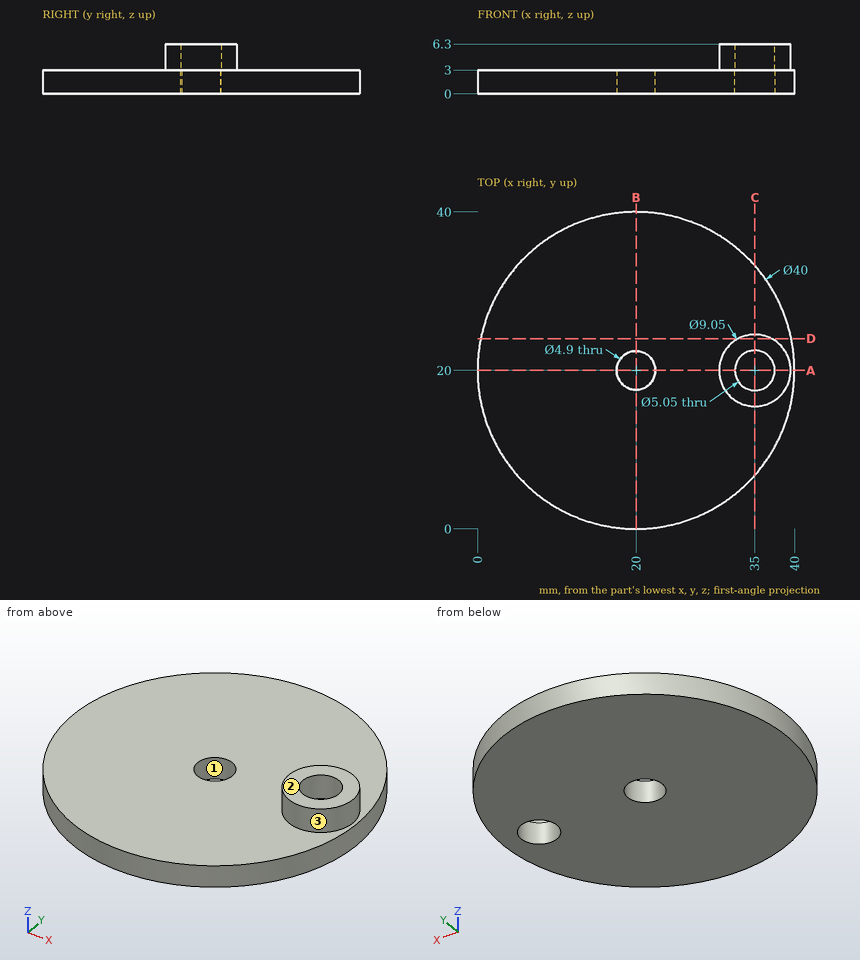
Source: three-view drawing plus pictorial views. Frame: mm from the lowest corner of the part. Give positions to 0.01 mm unless a question says otherwise; leave off trailing zeros. Write each loop counter-clockwise with the first axis right and the second up, starting at its lowest first coordinate (ties: lowest second). Pieces come first, ordered by that corner, then holes.
(1) First-contact query: P1, Ø2, axis at x = 9.5, z = 3, coming from the +Y side; P2, Ø2, axis at x = 6.5, z = 1, coming from the +Y side; P3, Ø2, axis at y = 20.5, z = 4.5, coming from the +X side (3 decimals). Flat tips, straight axial feed; report the tip coordinate or a pass-through.
(2) Cut plane B-B, the plane x = 20. Return loops of the section in (y, z).
(3) Cut plane A-A, the plane y = 20. Return loops of the section in (x, z) (3 decimals).
(4) Mould query, pull axis X, two halves, no side actions, for the marked faces 1, 2 and 3. Classes: released by +X, released by -X, zero draft, split by the parting line, or undercut.
(5) Ray query, line 1 (Y direction, x = 20, z = 1.6); line 2 (X direction, y = 18.5, z = 0.75); line 3 (Z direction, x = 33.5, y = 12.5). Return the intervals inside material, ascending.
(6) Cut plane C-C, the plane x = 35. Return loops of the section in (y, z) (3 decimals), then the cut area to 3 significant figures.
(7) Cut plane D-D, the plane y = 24. Return loops of the section in (x, z), then the cut area to 3 significant figures.
Values follow:
1. P1: stops at y = 37.6
1. P2: stops at y = 35.61
1. P3: stops at x = 39.525
2. outline: (0, 0) - (17.55, 0) - (17.55, 3) - (0, 3) - close; (22.45, 0) - (40, 0) - (40, 3) - (22.45, 3) - close
3. outline: (0, 0) - (17.55, 0) - (17.55, 3) - (0, 3) - close; (22.45, 0) - (32.475, 0) - (32.475, 6.3) - (30.475, 6.3) - (30.475, 3) - (22.45, 3) - close; (37.525, 0) - (40, 0) - (40, 3) - (39.525, 3) - (39.525, 6.3) - (37.525, 6.3) - close
4. face 1: undercut
4. face 2: zero draft
4. face 3: split by the parting line
5. line 1: y = 0 to 17.55, 22.45 to 40
5. line 2: x = 0.06 to 18.06, 21.94 to 32.97, 37.03 to 39.94
5. line 3: z = 0 to 3
6. outline: (6.771, 0) - (17.475, 0) - (17.475, 6.3) - (15.475, 6.3) - (15.475, 3) - (6.771, 3) - close; (22.525, 0) - (33.229, 0) - (33.229, 3) - (24.525, 3) - (24.525, 6.3) - (22.525, 6.3) - close
6. area: 77.4 mm2
7. outline: (0.4, 0) - (39.6, 0) - (39.6, 3) - (37.12, 3) - (37.12, 6.3) - (32.88, 6.3) - (32.88, 3) - (0.4, 3) - close
7. area: 132 mm2
